For this review, take the finished solid that the model builds, in its own axes (mm). A direction names the side the tool comes from. Give positions to 0.01 mm unless a question says otherwise; leave off trailing zeros. Order: outer loops, then holes, each group sorted by start corner. A loop starts at its lowest first (then second) coordinate and runs counter-clockwise, first axis right, second up.
Item 1: Consider section B-B (z = 77). Give the boundary of the cut face in (x, y), plus the area to 3 significant figures.
Item 2: Machinability: for faces 1 (the cylindrical face through (-1.32, 79.77, -29.97)), 2 (the cylindrical face through (103.504, 26.29, -0.198)), 3 (the flat face through (52.8, 11.5, -79.4)), 4 (the cylindrical face through (53.692, 66.738, -11.923)), which of the approach directions +Z, -Z, +X, -X, +Y, -Y give a long, thin tool a straight path to every point of the face, cutting with its end or side? Answer none if there is none.
Item 3: Consider section A-A (x = 108). Give the boundary of the cut face in (y, z), plus the area to 3 significant figures.
Item 4: For probe 1 along X at (y, z) = (73.75, 0); probe 2 along X at (y, z) = (21, 0); probe 3 along Z at (x, y) = (0, 16.25), list the stretches that pass through material, from the lowest coordinate up.
Item 5: Consider section D-D (y = 59.5). Give the boundary of the cut face in (x, z).
Item 6: The part is to be moulded in two halves that separate along X. For faces 5 (the cylindrical face through (-48.99, 58.2, 3.14)), 6 (the cylindrical face through (-12.465, 85.528, 39.584)), 7 (the flat face through (30, 70.5, 30)), say which applies: released by +X, released by -X, zero draft, split by the parting line, or undercut.
Item 7: Consider section C-C (x = 69.5). Give the boundary of the cut face in (y, z).
Item 8: For P1, Ø1.5, axis at x = 22.5, y = 49.5, coming from the -Z side; P2, Ø3, axis at x = 58, z = 42, coming from the +Y side; P3, Ø0.6, axis at y = 48.5, z = -1, coming from the +X side; P4, Ø5.5, axis at x = -54, z = 93.53, coming from the -Y side, all flat-tipped, find the tip position at first contact; note any pin that passes through.
```python
from build123d import *

# Parameters (mm, degrees)
SKETCH_3_R              = 1
CUT_EXTRUDE_1_DEPTH     = 184.766835963
SKETCH_4_W              = 12
SKETCH_4_H              = 2
HOLE_WIZARD_M8_1_REACH  = 230.003
HOLE_WIZARD_M8_1_BORE_R = 3.4
HOLE_START              = 11.5
HOLE_WIZARD_2_OUTLINE_R = 4.5
HOLE_WIZARD_2_DEPTH     = 30


# Read off the part's stored shape, not the designer's step: 孔2
with BuildPart() as part:
    # 草图1 → 旋转1 (revolve)
    with BuildSketch(Plane(origin=(0, 0, 0), x_dir=(0, 0, -1), z_dir=(1, 0, 0))):
        with BuildLine():
            Line((0, 0), (-99, 0))
            Line((-99, 0), (-99, 3.5))
            Line((-99, 3.5), (-95, 3.5))
            Line((-95, 3.5), (-95, 11.5))
            Line((-95, 11.5), (-120, 11.5))
            Line((-120, 11.5), (-120, 41.5))
            Line((-120, 41.5), (-63, 41.5))
            ThreePointArc((-63, 41.5), (-57.343145751, 43.843145751), (-55, 49.5))
            Line((-55, 49.5), (-55, 83.5))
            Line((-55, 83.5), (-41.5, 83.5))
            Line((-41.5, 83.5), (-41.5, 87.5))
            Line((-41.5, 87.5), (0, 87.5))
            Line((0, 87.5), (0, 0))
        make_face()
    revolve(axis=Axis((0, 87.5, 0), (0, -1, 0)))

    # 草图2 → 切除-旋转1 (revolve, cut)
    with BuildSketch(Plane(origin=(0, 0, 0), x_dir=(0, 0, -1), z_dir=(1, 0, 0))):
        Polygon((-89, 0), (-89, 29), (-55, 29), (-45, 46.320508076), (-45, 70.5), (-42, 70.5), (-42, 72), (-36, 72), (-36, 78.5), (-30, 78.5), (-30, 81), (-25.5, 81), (-25.5, 87.5), (0, 87.5), (0, 0), align=None)
    revolve(axis=Axis((0, 87.5, 0), (0, -1, 0)), mode=Mode.SUBTRACT)

    # 草图3 → 切除-拉伸1 (cut, through all)
    with BuildSketch(Plane.XZ.offset(-70.5)):
        with Locations((-45, 0)):
            Circle(SKETCH_3_R)
    extrude(amount=CUT_EXTRUDE_1_DEPTH, mode=Mode.SUBTRACT)

    # 草图4 → 孔1 (revolve, cut)
    with BuildSketch(Plane(origin=(-55, 59.5, 0), x_dir=(0, 0, 1), z_dir=(0, 1, 0))):
        with Locations((6, 1)):
            Rectangle(SKETCH_4_W, SKETCH_4_H)
    revolve(axis=Axis((55, 59.5, 0), (-1, 0, 0)), mode=Mode.SUBTRACT)

    # M8 螺纹孔1 bore → M8 螺纹孔1 (cut, up to next)
    with BuildSketch(Plane.ZY.offset(53), mode=Mode.PRIVATE) as hole_wizard_m8_1_sk1:
        with Locations((0, 59.5)):
            Circle(HOLE_WIZARD_M8_1_BORE_R)
    hole_wizard_m8_1_tool1 = extrude(hole_wizard_m8_1_sk1.sketch, amount=-HOLE_WIZARD_M8_1_REACH, mode=Mode.PRIVATE) & part.part
    add(hole_wizard_m8_1_tool1.solids().sort_by_distance((-53, 59.5, 0))[0], mode=Mode.SUBTRACT)

    # 孔2 outline → 孔2 (cut)
    with BuildSketch(Plane(origin=(0, 0, 0), x_dir=(1, 0, 0), z_dir=(0, 1, 0)).offset(HOLE_START)):
        with Locations((-54, 93.530743609)):
            Circle(HOLE_WIZARD_2_OUTLINE_R)
        with Locations((54, 93.530743609)):
            Circle(HOLE_WIZARD_2_OUTLINE_R)
        with Locations((108, 0)):
            Circle(HOLE_WIZARD_2_OUTLINE_R)
        with Locations((54, -93.530743609)):
            Circle(HOLE_WIZARD_2_OUTLINE_R)
        with Locations((-54, -93.530743609)):
            Circle(HOLE_WIZARD_2_OUTLINE_R)
        with Locations((-108, 0)):
            Circle(HOLE_WIZARD_2_OUTLINE_R)
    extrude(amount=HOLE_WIZARD_2_DEPTH, mode=Mode.SUBTRACT)


solid = part.part
```
Resolved:
1. outline: (-92.04, 11.5) - (-55.64, 11.5) - (-55.64, 3.5) - (-62.23, 3.5) - (-62.23, 0) - (-44.63, 0) - (-44.63, 29) - (44.63, 29) - (44.63, 0) - (62.23, 0) - (62.23, 3.5) - (55.64, 3.5) - (55.64, 11.5) - (92.04, 11.5) - (92.04, 41.5) - (-92.04, 41.5) - close
1. area: 4,260 mm2
2. face 1: -Y
2. face 2: +Y, -Y
2. face 3: none
2. face 4: +Y
3. outline: (11.5, -52.31) - (41.5, -52.31) - (41.5, -4.5) - (11.5, -4.5) - close; (11.5, 4.5) - (41.5, 4.5) - (41.5, 52.31) - (11.5, 52.31) - close
3. area: 2,870 mm2
4. probe 1: x = -55 to -36, 36 to 55
4. probe 2: x = -120 to -112.5, -103.5 to -89, 89 to 103.5, 112.5 to 120
4. probe 3: z = -120 to -89, 89 to 120
5. outline: (-53.67, -12) arc R55 ccw (long way) to (-53.67, 12) - (-53, 12) - (-53, 3.4) - (-44.87, 3.4) arc R45 cw (long way) to (-44.87, -3.4) - (-53, -3.4) - (-53, -12) - close
6. face 5: zero draft
6. face 6: split by the parting line
6. face 7: undercut
7. outline: (0, -70.5) - (3.5, -70.5) - (3.5, -64.77) - (11.5, -64.77) - (11.5, -97.83) - (41.5, -97.83) - (41.5, 97.83) - (11.5, 97.83) - (11.5, 64.77) - (3.5, 64.77) - (3.5, 70.5) - (0, 70.5) - (0, 55.59) - (29, 55.59) - (29, -55.59) - (0, -55.59) - close
8. P1: stops at z = -50.52
8. P2: stops at y = 41.5
8. P3: stops at x = 55.1
8. P4: passes through
